```python
from build123d import *

# Parameters (mm, degrees)
SKETCH1_W           = 420
SKETCH1_H           = 110
BOSS_EXTRUDE1_DEPTH = 2
SKETCH2_W           = 100
SKETCH2_H           = 4.4
CUT_EXTRUDE1_DEPTH  = 2
FILLET1_R           = 1.5
CUT_EXTRUDE2_REACH  = 4
SKETCH3_R           = 3
CUT_EXTRUDE3_REACH  = 4
SKETCH4_R           = 3
SKETCH4_R_2         = 8.25


with BuildPart() as part:
    # Sketch1 → Boss-Extrude1 (new body)
    with BuildSketch(Plane(origin=(23.948254466, 0, 0), x_dir=(0, 0, -1), z_dir=(1, 0, 0))):
        with Locations((-184.692172039, 45)):
            Rectangle(SKETCH1_W, SKETCH1_H)
    extrude(amount=BOSS_EXTRUDE1_DEPTH)

    # Sketch2 → Cut-Extrude1 (cut)
    with BuildSketch(Plane(origin=(25.948254466, 0, 0), x_dir=(0, 0, -1), z_dir=(1, 0, 0))):
        with Locations((-314.692172039, 54.3)):
            Rectangle(SKETCH2_W, SKETCH2_H)
        with Locations((-314.692172039, 38.3)):
            Rectangle(SKETCH2_W, SKETCH2_H)
        with Locations((-114.692172039, 54.3)):
            Rectangle(SKETCH2_W, SKETCH2_H)
        with Locations((-114.692172039, 38.3)):
            Rectangle(SKETCH2_W, SKETCH2_H)
    extrude(amount=-CUT_EXTRUDE1_DEPTH, mode=Mode.SUBTRACT)

    # Fillet1
    fillet1_edges = [part.edges().sort_by_distance(p)[0] for p in [
        (24.948254466, 52.1, 364.692172039),
        (24.948254466, 56.5, 364.692172039),
        (24.948254466, 56.5, 264.692172039),
        (24.948254466, 52.1, 264.692172039),
        (24.948254466, 36.1, 364.692172039),
        (24.948254466, 40.5, 364.692172039),
        (24.948254466, 40.5, 264.692172039),
        (24.948254466, 36.1, 264.692172039),
        (24.948254466, 56.5, 64.692172039),
        (24.948254466, 52.1, 64.692172039),
        (24.948254466, 52.1, 164.692172039),
        (24.948254466, 56.5, 164.692172039),
        (24.948254466, 36.1, 164.692172039),
        (24.948254466, 40.5, 164.692172039),
        (24.948254466, 40.5, 64.692172039),
        (24.948254466, 36.1, 64.692172039),
    ]]
    fillet(fillet1_edges, radius=FILLET1_R)

    # Sketch3 → Cut-Extrude2 (cut, up to next)
    with BuildSketch(Plane(origin=(25.948254466, 0, 0), x_dir=(0, 0, -1), z_dir=(1, 0, 0)), mode=Mode.PRIVATE) as cut_extrude2_sk1:
        with Locations((-389.692172039, 75)):
            Circle(SKETCH3_R)
    cut_extrude2_tool1 = extrude(cut_extrude2_sk1.sketch, amount=-CUT_EXTRUDE2_REACH, mode=Mode.PRIVATE) & part.part
    add(cut_extrude2_tool1.solids().sort_by_distance((25.948254, 75, 389.692172))[0], mode=Mode.SUBTRACT)
    # Sketch3 → Cut-Extrude2 (cut, up to next)
    with BuildSketch(Plane(origin=(25.948254466, 0, 0), x_dir=(0, 0, -1), z_dir=(1, 0, 0)), mode=Mode.PRIVATE) as cut_extrude2_sk2:
        with Locations((-389.692172039, 25)):
            Circle(SKETCH3_R)
    cut_extrude2_tool2 = extrude(cut_extrude2_sk2.sketch, amount=-CUT_EXTRUDE2_REACH, mode=Mode.PRIVATE) & part.part
    add(cut_extrude2_tool2.solids().sort_by_distance((25.948254, 25, 389.692172))[0], mode=Mode.SUBTRACT)
    # Sketch3 → Cut-Extrude2 (cut, up to next)
    with BuildSketch(Plane(origin=(25.948254466, 0, 0), x_dir=(0, 0, -1), z_dir=(1, 0, 0)), mode=Mode.PRIVATE) as cut_extrude2_sk3:
        with Locations((20.307827961, 75)):
            Circle(SKETCH3_R)
    cut_extrude2_tool3 = extrude(cut_extrude2_sk3.sketch, amount=-CUT_EXTRUDE2_REACH, mode=Mode.PRIVATE) & part.part
    add(cut_extrude2_tool3.solids().sort_by_distance((25.948254, 75, -20.307828))[0], mode=Mode.SUBTRACT)
    # Sketch3 → Cut-Extrude2 (cut, up to next)
    with BuildSketch(Plane(origin=(25.948254466, 0, 0), x_dir=(0, 0, -1), z_dir=(1, 0, 0)), mode=Mode.PRIVATE) as cut_extrude2_sk4:
        with Locations((20.307827961, 25)):
            Circle(SKETCH3_R)
    cut_extrude2_tool4 = extrude(cut_extrude2_sk4.sketch, amount=-CUT_EXTRUDE2_REACH, mode=Mode.PRIVATE) & part.part
    add(cut_extrude2_tool4.solids().sort_by_distance((25.948254, 25, -20.307828))[0], mode=Mode.SUBTRACT)

    # Sketch4 → Cut-Extrude3 (cut, up to next)
    with BuildSketch(Plane(origin=(25.948254466, 0, 0), x_dir=(0, 0, -1), z_dir=(1, 0, 0)), mode=Mode.PRIVATE) as cut_extrude3_sk1:
        with Locations((-274.692172039, 10)):
            Circle(SKETCH4_R)
    cut_extrude3_tool1 = extrude(cut_extrude3_sk1.sketch, amount=-CUT_EXTRUDE3_REACH, mode=Mode.PRIVATE) & part.part
    add(cut_extrude3_tool1.solids().sort_by_distance((25.948254, 10, 274.692172))[0], mode=Mode.SUBTRACT)
    # Sketch4 → Cut-Extrude3 (cut, up to next)
    with BuildSketch(Plane(origin=(25.948254466, 0, 0), x_dir=(0, 0, -1), z_dir=(1, 0, 0)), mode=Mode.PRIVATE) as cut_extrude3_sk2:
        with Locations((-94.692172039, 10)):
            Circle(SKETCH4_R)
    cut_extrude3_tool2 = extrude(cut_extrude3_sk2.sketch, amount=-CUT_EXTRUDE3_REACH, mode=Mode.PRIVATE) & part.part
    add(cut_extrude3_tool2.solids().sort_by_distance((25.948254, 10, 94.692172))[0], mode=Mode.SUBTRACT)
    # Sketch4 → Cut-Extrude3 (cut, up to next)
    with BuildSketch(Plane(origin=(25.948254466, 0, 0), x_dir=(0, 0, -1), z_dir=(1, 0, 0)), mode=Mode.PRIVATE) as cut_extrude3_sk3:
        with Locations((-44.692172039, 44.3)):
            Circle(SKETCH4_R_2)
    cut_extrude3_tool3 = extrude(cut_extrude3_sk3.sketch, amount=-CUT_EXTRUDE3_REACH, mode=Mode.PRIVATE) & part.part
    add(cut_extrude3_tool3.solids().sort_by_distance((25.948254, 44.3, 44.692172))[0], mode=Mode.SUBTRACT)
    # Sketch4 → Cut-Extrude3 (cut, up to next)
    with BuildSketch(Plane(origin=(25.948254466, 0, 0), x_dir=(0, 0, -1), z_dir=(1, 0, 0)), mode=Mode.PRIVATE) as cut_extrude3_sk4:
        with Locations((-274.692172039, 80)):
            Circle(SKETCH4_R)
    cut_extrude3_tool4 = extrude(cut_extrude3_sk4.sketch, amount=-CUT_EXTRUDE3_REACH, mode=Mode.PRIVATE) & part.part
    add(cut_extrude3_tool4.solids().sort_by_distance((25.948254, 80, 274.692172))[0], mode=Mode.SUBTRACT)
    # Sketch4 → Cut-Extrude3 (cut, up to next)
    with BuildSketch(Plane(origin=(25.948254466, 0, 0), x_dir=(0, 0, -1), z_dir=(1, 0, 0)), mode=Mode.PRIVATE) as cut_extrude3_sk5:
        with Locations((-94.692172039, 80)):
            Circle(SKETCH4_R)
    cut_extrude3_tool5 = extrude(cut_extrude3_sk5.sketch, amount=-CUT_EXTRUDE3_REACH, mode=Mode.PRIVATE) & part.part
    add(cut_extrude3_tool5.solids().sort_by_distance((25.948254, 80, 94.692172))[0], mode=Mode.SUBTRACT)


solid = part.part
```
Input: part model. Units: mm. Frame: model coordinates. Coordinates: 2 decimals unless noted, no trailing zeros. Write each loop counter-clockwise with the first axis right and the second up, starting at its lowest first coordinate (ties: lowest second). Pieces come first, ordered by that corner, then holes. Notation, with made-up numbers: M 40.5,39.5 L 96.5,39.5 A15 cw 96.5,49.5 Z; hole C 12,-6 d2. An arc over 180 degrees is marked long. Use one line per item in the form item = value.
Q1. Section A-A (z = 76). Return loops of the section in (x, y), plus the area to 3 significant figures.
Answer below:
outline = M 23.95,-10 L 25.95,-10 L 25.95,36.1 L 23.95,36.1 Z; M 23.95,40.5 L 25.95,40.5 L 25.95,52.1 L 23.95,52.1 Z; M 23.95,56.5 L 25.95,56.5 L 25.95,100 L 23.95,100 Z
area = 202 mm²
Q2. Draft query along Z for faces 1 (the face through (24.96, 39.28, 51.24)), 2 (the face through (23.948, 46, 188)). Return one class per face: released by +Z, released by -Z, zero draft, split by the parting line, or undercut.
Answer below:
face_1 = undercut
face_2 = zero draft
Q3. Section B-B (y = 44.3). Return loops of the section in (x, z), plus the area to 3 significant figures.
Answer below:
outline = M 23.95,-25.31 L 25.95,-25.31 L 25.95,36.44 L 23.95,36.44 Z; M 23.95,52.94 L 25.95,52.94 L 25.95,394.69 L 23.95,394.69 Z
area = 807 mm²
Q4. Section C-C (x = 25.4). Count the separate pieces of the cut face and the enclosed holes in it, plus the area to 3 significant figures.
Answer below:
separate_pieces = 1
enclosed_holes = 13
area = 44,000 mm²
Q5. Material intervals for probe 1 along Y at (x, z) = (25, 288.5); probe 2 along Z at (x, y) = (24.7, 11), sorted ascending. Write a range as from..to.
Answer below:
probe_1 = -10..36.1, 40.5..52.1, 56.5..100
probe_2 = -25.31..91.86, 97.52..271.86, 277.52..394.69
